```python
from build123d import *

# Parameters (mm, degrees)
BOSS_EXTRUDE1_DEPTH = 122
SKETCH3_W           = 60.039506293
SKETCH3_H           = 115
CUT_EXTRUDE1_DEPTH  = 122
BOSS_EXTRUDE3_DEPTH = 116.5
BOSS_EXTRUDE4_DEPTH = 116.5
BOSS_EXTRUDE5_DEPTH = 116.5
SKETCH10_W          = 63
SKETCH10_H          = 2
BOSS_EXTRUDE6_DEPTH = 5


with BuildPart() as part:
    # Sketch1 → Boss-Extrude1 (new body)
    with BuildSketch(Plane.XY):
        Polygon((0, 0), (67, 0), (0, 38), align=None)
    extrude(amount=BOSS_EXTRUDE1_DEPTH)

    # Sketch3 → Cut-Extrude1 (cut)
    with BuildSketch(Plane.XZ):
        with Locations((33.519753147, 61)):
            Rectangle(SKETCH3_W, SKETCH3_H)
    extrude(amount=-CUT_EXTRUDE1_DEPTH, mode=Mode.SUBTRACT)

    # Sketch4 → Boss-Extrude3 (add)
    with BuildSketch(Plane(origin=(0, 0, 118.5), x_dir=(-1, 0, 0), z_dir=(0, 0, -1))):
        Polygon((-3.5, 33.514925373), (-3.5, 30.640822028), (-57.429863124, 0.05373548), (-57.429863124, 2.927838825), align=None)
    extrude(amount=BOSS_EXTRUDE3_DEPTH)

    # Sketch6 → Boss-Extrude4 (add)
    with BuildSketch(Plane(origin=(0, 0, 118.5), x_dir=(-1, 0, 0), z_dir=(0, 0, -1))):
        Polygon((-57.429863124, 2.927838825), (-58.502676203, 4.819377676), (-63.539506293, 1.962668073), (-63.539506293, 0), (-57.429863124, 0.05373548), align=None)
    extrude(amount=BOSS_EXTRUDE4_DEPTH)

    # Sketch9 → Boss-Extrude5 (add)
    with BuildSketch(Plane.XY.offset(3.5)):
        Polygon((58.502676203, 4.819377676), (57.502676203, 5.386541855), (56.429863124, 3.495003005), (57.429863124, 2.927838825), align=None)
    extrude(amount=BOSS_EXTRUDE5_DEPTH)

    # Sketch10 → Boss-Extrude6 (add)
    with BuildSketch(Plane.XZ):
        Polygon((0, 122), (0, 0), (2, 0), (2, 2), (2, 120), (2, 122), align=None)
        Polygon((67, 122), (2, 122), (2, 120), (65, 120), (67, 120), align=None)
        with Locations((33.5, 1)):
            Rectangle(SKETCH10_W, SKETCH10_H)
        Polygon((65, 2), (65, 0), (67, 0), (67, 120), (65, 120), align=None)
    extrude(amount=BOSS_EXTRUDE6_DEPTH)


solid = part.part
```
For this review, take the finished solid that the model builds, in its own axes (mm). A direction names the side the tool comes from. Round coordinates to 2 decimals unless told otherwise and drop trailing zeros. Loops run counter-clockwise (first coordinate to the right, second up) from the corner with the lowest first, then second, coordinate; pieces in that order, holes last.
Q1. To check wall thickness, follow line 1 along Z through (x, y) = (49, 10); line 2 along X through (y, z) = (36, 83); line 3 along X through (y, z) = (14.5, 96). State the ranges of each line that lie inside material, in increasing order.
Result sheet:
line 1: z = 0 to 3.5, 118.5 to 122
line 2: x = 0 to 3.5
line 3: x = 0 to 3.5, 31.96 to 37.03
Q2. Mouldability with a two-part tool opening along Z and no side actions: class faces 4 (the face through (27, 12, 122)), 5 (the face through (30.34, 18.29, 61.8)), 6 (the face through (67, -2, 60)) as +Z half, -Z half, draft (parallel to the pull), parting line (faces both ways), or undercut.
Result sheet:
face 4: +Z half
face 5: undercut
face 6: draft
Q3. Add section A-A on y = 19. Write out the cut boundary in (x, z), plus the area to 3 significant figures.
Result sheet:
outline: (0, 0) - (33.5, 0) - (33.5, 3.5) - (29.09, 3.5) - (29.09, 118.5) - (33.5, 118.5) - (33.5, 122) - (0, 122) - close; hole (3.5, 3.5) - (24.02, 3.5) - (24.02, 118.5) - (3.5, 118.5) - close
area: 1,220 mm2
Q4. Machinability: for faces 1 (the face through (0, 17, 62)), 2 (the face through (30.09, 15.56, 61.8)), 3 (the face through (3.5, 35, 60)), which of the approach directions +Z, -Z, +X, -X, +Y, -Y give a long, thin tool a straight path to every point of the face, cutting with its end or side? Answer none if there is none.
Result sheet:
face 1: +Z, -Z, -X, +Y, -Y
face 2: -Y
face 3: +X, +Y
Q5. Insertion check: pin 1 Ø9 at (y, z) = (10.5, 72.5) entering from +X; pin 2 Ø6 at (x, z) = (52, 29) entering from +Y; pin 3 Ø8 at (x, z) = (21.5, 31.5) entering from +Y. Each pin has a flat end and moves straight along its axis. Give the tip position at first contact, or say it passes through.
Result sheet:
pin 1: stops at x = 52.01
pin 2: stops at y = 7.71
pin 3: stops at y = 25.57
Q6. Add section B-B on z = 60. Write out the cut boundary in (x, y) (1 decimal).
Result sheet:
outline: (0, -5) - (2, -5) - (2, 0) - (3.5, 0) - (3.5, 30.6) - (57.4, 0.1) - (63.5, 0) - (65, 0) - (65, -5) - (67, -5) - (67, 0) - (57.5, 5.4) - (56.4, 3.5) - (3.5, 33.5) - (3.5, 36) - (0, 38) - close
Q7. Add section D-D on y = 12. Write out the cut boundary in (x, z).
Result sheet:
outline: (0, 0) - (45.84, 0) - (45.84, 3.5) - (41.43, 3.5) - (41.43, 118.5) - (45.84, 118.5) - (45.84, 122) - (0, 122) - close; hole (3.5, 3.5) - (36.37, 3.5) - (36.37, 118.5) - (3.5, 118.5) - close
Q8. Add section C-C on x = 50.5. Write out the cut boundary in (y, z).
Result sheet:
outline: (-5, 0) - (9.36, 0) - (9.36, 3.5) - (6.86, 3.5) - (6.86, 118.5) - (9.36, 118.5) - (9.36, 122) - (-5, 122) - (-5, 120) - (0, 120) - (0, 118.5) - (3.98, 118.5) - (3.98, 3.5) - (0, 3.5) - (0, 2) - (-5, 2) - close
